```python
from build123d import *

# Parameters (mm, degrees)
BOSS_EXTRUDE1_DEPTH     = 33.02
BOSS_EXTRUDE2_START     = 6.35
BOSS_EXTRUDE2_DEPTH     = 6.35
CUT_EXTRUDE1_DEPTH      = 96.52
CUT_EXTRUDE1_DEPTH_BACK = 96.52
SKETCH3_W               = 90.275574195
SKETCH3_H               = 26.596699
SKETCH3_W_2             = 48.373898049


with BuildPart() as part:
    # Sketch1 → Boss-Extrude1 (new body)
    with BuildSketch(Plane(origin=(0, 0, 0), x_dir=(1, 0, 0), z_dir=(0, 1, 0))):
        with BuildLine():
            Line((-22.221083262, 74.846156038), (-22.221083262, 50.8))
            Line((-22.221083262, 50.8), (-21.932164151, 48.906379538))
            Line((-21.932164151, 48.906379538), (-4.668805876, -6.35))
            Line((-4.668805876, -6.35), (87.218118757, -6.35))
            Line((87.218118757, -6.35), (104.489731546, 48.905528077))
            ThreePointArc((104.489731546, 48.905528077), (104.706204131, 49.841791784), (104.778916738, 50.8))
            Line((104.778916738, 50.8), (104.778916738, 74.846156038))
            Line((104.778916738, 74.846156038), (72.957581245, 125.760292827))
            Line((72.957581245, 125.760292827), (69.402851201, 215.965853579))
            ThreePointArc((69.402851201, 215.965853579), (41.278916738, 244.089788041), (13.154982275, 215.965853579))
            Line((13.154982275, 215.965853579), (9.600252232, 125.760292827))
            Line((9.600252232, 125.760292827), (-22.221083262, 74.846156038))
        make_face()
        with BuildLine():
            Line((82.55, 0), (0, 0))
            Line((0, 0), (-15.871083262, 50.8))
            Line((-15.871083262, 50.8), (-15.871083262, 73.025))
            Line((-15.871083262, 73.025), (15.878916738, 123.825))
            Line((15.878916738, 123.825), (19.500057517, 215.715813233))
            ThreePointArc((19.500057517, 215.715813233), (41.278916738, 237.494672454), (63.057775959, 215.715813233))
            Line((63.057775959, 215.715813233), (66.678916738, 123.825))
            Line((66.678916738, 123.825), (98.428916738, 73.025))
            Line((98.428916738, 73.025), (98.428916738, 50.8))
            Line((98.428916738, 50.8), (82.55, 0))
        make_face(mode=Mode.SUBTRACT)
    extrude(amount=BOSS_EXTRUDE1_DEPTH)

    # Sketch2 → Boss-Extrude2 (add)
    # profile 1 of 2: a face of its own
    with BuildSketch(Plane.XZ.offset(BOSS_EXTRUDE2_START)):
        with BuildLine():
            Line((104.706204131, -49.841791784), (104.778916738, -50.8))
            Line((104.778916738, -50.8), (104.778916738, -74.846156038))
            Line((104.778916738, -74.846156038), (72.957581245, -125.760292827))
            Line((72.957581245, -125.760292827), (69.402851201, -215.965853579))
            ThreePointArc((69.402851201, -215.965853579), (41.278916738, -244.089788041), (13.154982275, -215.965853579))
            Line((13.154982275, -215.965853579), (9.600252232, -125.760292827))
            Line((9.600252232, -125.760292827), (-22.221083262, -74.846156038))
            Line((-22.221083262, -74.846156038), (-22.221083262, -50.8))
            Line((-22.221083262, -50.8), (-21.932164151, -48.906379538))
            Line((-21.932164151, -48.906379538), (-4.668805876, 6.35))
            Line((-4.668805876, 6.35), (87.218118757, 6.35))
            Line((87.218118757, 6.35), (104.489731546, -48.905528077))
            Line((104.489731546, -48.905528077), (104.706204131, -49.841791784))
        make_face()
        with BuildLine():
            Line((66.678916738, -123.825), (63.057775959, -215.715813233))
            ThreePointArc((63.057775959, -215.715813233), (41.278916738, -237.494672454), (19.500057517, -215.715813233))
            Line((19.500057517, -215.715813233), (15.878916738, -123.825))
            Line((15.878916738, -123.825), (-15.871083262, -73.025))
            Line((-15.871083262, -73.025), (-15.871083262, -50.8))
            Line((-15.871083262, -50.8), (0, 0))
            Line((0, 0), (82.55, 0))
            Line((82.55, 0), (98.428916738, -50.8))
            Line((98.428916738, -50.8), (98.428916738, -73.025))
            Line((98.428916738, -73.025), (66.678916738, -123.825))
        make_face(mode=Mode.SUBTRACT)
    # profile 2 of 2: a face of its own
    with BuildSketch(Plane.XZ.offset(BOSS_EXTRUDE2_START)):
        with BuildLine():
            ThreePointArc((63.057775959, -215.715813233), (41.278916738, -237.494672454), (19.500057517, -215.715813233))
            Line((19.500057517, -215.715813233), (15.878916738, -123.825))
            Line((15.878916738, -123.825), (-15.871083262, -73.025))
            Line((-15.871083262, -73.025), (-15.871083262, -50.8))
            Line((-15.871083262, -50.8), (0, 0))
            Line((0, 0), (82.55, 0))
            Line((82.55, 0), (98.428916738, -50.8))
            Line((98.428916738, -50.8), (98.428916738, -73.025))
            Line((98.428916738, -73.025), (66.678916738, -123.825))
            Line((66.678916738, -123.825), (63.057775959, -215.715813233))
        make_face()
    extrude(amount=-BOSS_EXTRUDE2_DEPTH)

    # Sketch3 → Cut-Extrude1 (cut, two sides: drawn at the far end of the back side and taken through both)
    with BuildSketch(Plane(origin=(4.637215869, 0, 0.182738741), x_dir=(-0.03937643239096595, 0, 0.9992244475452748), z_dir=(-0.9992244475452748, 0, -0.03937643239096595)).offset(-CUT_EXTRUDE1_DEPTH_BACK)):
        with Locations((-171.178569904, 13.2983495)):
            Rectangle(SKETCH3_W, SKETCH3_H)
        with Locations((-240.503306026, 13.2983495)):
            Rectangle(SKETCH3_W_2, SKETCH3_H)
    extrude(amount=CUT_EXTRUDE1_DEPTH + CUT_EXTRUDE1_DEPTH_BACK, mode=Mode.SUBTRACT)


solid = part.part
```
The listing builds one solid part. Answer for the finished solid, in the listing's coordinates (mm). A direction names the side the tool comes from. Give positions to 0.01 mm unless a question says otherwise; leave off trailing zeros. Order: outer loops, then holes, each group sorted by start corner. A loop starts at its lowest first (then second) coordinate and runs counter-clockwise, first axis right, second up. Notation, with made-up numbers: (31, 75.25) -> (65, 75.25) arc R9 cw to (65, 90.25) -> close; hole circle Ø6 at (42.5, 82.25). An arc over 180 degrees is marked (long way). One line per item, written item: value.
1) Determine the mould class of faces 1 (the cylindrical face through (41.897, -3.219, -244.083)), 2 (the flat face through (42, 16, 0)), 3 (the flat face through (70.77, 13.11, -123.35)) for opening direction X: pulls with the +X half, pulls with the -X half, needs draft (parallel to the pull), parting line crosses it, or undercut.
Reported:
face 1: parting line crosses it
face 2: undercut
face 3: pulls with the +X half
2) Find section B-B, the plane x = 58.5. Determine the outline of the cut face in (y, z).
Reported:
outline: (-6.35, -238.2) -> (0, -238.2) -> (0, 0) -> (33.02, 0) -> (33.02, 6.35) -> (-6.35, 6.35) -> close; (26.6, -238.2) -> (33.02, -238.2) -> (33.02, -229.05) -> (26.6, -229.05) -> close
3) Find section A-A, the plane z = -143. Determine the outline of the cut face in (x, y).
Reported:
outline: (10.28, -6.35) -> (72.28, -6.35) -> (72.28, 0) -> (10.28, 0) -> close; (10.28, 26.6) -> (16.63, 26.6) -> (16.63, 33.02) -> (10.28, 33.02) -> close; (65.92, 26.6) -> (72.28, 26.6) -> (72.28, 33.02) -> (65.92, 33.02) -> close
4) Find section D-D, the plane y = 2.5. Determine the outline of the cut face in (x, z) (3 decimals), plus the area to 3 significant figures.
Reported:
outline: (-22.221, -74.846) -> (9.6, -125.76) -> (15.945, -125.51) -> (15.879, -123.825) -> (-15.871, -73.025) -> (-15.871, -50.8) -> (0, 0) -> (82.55, 0) -> (98.429, -50.8) -> (98.429, -73.025) -> (66.88, -123.503) -> (74.557, -123.201) -> (104.779, -74.846) -> (104.779, -50.8) arc R6.35 ccw to (104.49, -48.906) -> (87.218, 6.35) -> (-4.669, 6.35) -> (-21.932, -48.906) -> (-22.221, -50.8) -> close
area: 2,320 mm^2
5) A tool of negligible diameter and unlimited length cuts with its end or side. For faces 4 (the flat face through (12.817, 13.112, -125.634)), 5 (the flat face through (82.33, 16.28, -98.78)), 6 (the flat face through (12.8, 33.02, -119.5)), from which of +Z, -Z, +X, -X, +Y, -Y can it reach the whole face along a straight path? Write none if from no direction.
Reported:
face 4: -Z, +X
face 5: +Y
face 6: +Z, -Z, +X, -X, +Y
6) Flat-ended cylindrical pins translate along their axes: P1, Ø5, axis at y = 6.5, z = -40.5, coming from the +X side; P2, Ø2, axis at x = 86.5, z = -107, coming from the -Y side; P3, Ø3, axis at x = 75.5, y = 15.5, coming from the -Z side; P4, Ø12, axis at x = 65, y = 0.5, coming from the -Z side. Find the tip coordinate at first contact, or state that the pin passes through.
Reported:
P1: stops at x = 102.64
P2: passes through
P3: stops at z = -123.22
P4: stops at z = -237.79
7) Find section C-C, the plane z = -56.5. Determine the outline of the cut face in (x, y), plus the area to 3 significant figures.
Reported:
outline: (-22.22, -6.35) -> (104.78, -6.35) -> (104.78, 33.02) -> (98.43, 33.02) -> (98.43, 0) -> (-15.87, 0) -> (-15.87, 33.02) -> (-22.22, 33.02) -> close
area: 1,230 mm^2
8) Find the intervals of material crossed by line 1 (X direction, y = 16.5, z = -64); line 2 (Y direction, x = 47.5, z = -204); line 3 (X direction, y = 24, z = -11.5), in increasing order.
Reported:
line 1: x = -22.22 to -15.87, 98.43 to 104.78
line 2: y = -6.35 to 0
line 3: x = -10.25 to -3.59, 86.14 to 92.8
